Design review of the part built by this model. Coordinates are the model's own, in mm. Coordinates: 2 decimals unless noted, no trailing zeros. Loops run counter-clockwise (first coordinate to the right, second up) from the corner with the lowest first, then second, coordinate; pieces in that order, holes last. Notation, with made-up numbers: M 48,13.25 L 67,13.25 A29 ccw 67,40.25 Z; hole C 83,76 d4. An arc over 180 degrees is marked long. Write item = value, one per line. Start each with the question number.
```python
from build123d import *

# Parameters (mm, degrees)
SKETCH2_R           = 11.1125
BOSS_EXTRUDE1_DEPTH = 3.175
FILLET1_R           = 3
FILLET2_R           = 1


with BuildPart() as part:
    # Sketch2 → Boss-Extrude1 (new body)
    with BuildSketch(Plane.XY):
        with BuildLine():
            Line((-364.964629933, 19.05), (-397.035370067, 19.05))
            Line((-397.035370067, 19.05), (-397.035370067, -34.925))
            Line((-397.035370067, -34.925), (-520.207659615, -112.081032385))
            Line((-520.207659615, -112.081032385), (-530.464644327, -134.880029394))
            add(Edge.make_bspline(
                [(-457.420545856, -119.022880851), (-481.278146928, -107.716723517), (-513.288827873, -114.168548124), (-530.464644327, -134.880029394)],
                knots=[0.042886926, 0.042886926, 0.042886926, 0.042886926, 1, 1, 1, 1], degree=3))
            Line((-457.420545856, -119.022880851), (-364.964629933, -24.022670771))
            Line((-364.964629933, -24.022670771), (-364.964629933, 19.05))
        make_face()
        with Locations((-381, 0)):
            Circle(SKETCH2_R, mode=Mode.SUBTRACT)
    extrude(amount=BOSS_EXTRUDE1_DEPTH)

    # Fillet1
    fillet1_edges = [part.edges().sort_by_distance(p)[0] for p in [
        (-520.207659615, -112.081032385, 1.5875),
        (-397.035370067, -34.925, 1.5875),
        (-457.420545856, -119.022880851, 1.5875),
        (-364.964629933, -24.022670771, 1.5875),
        (-397.035370067, 19.05, 1.5875),
        (-364.964629933, 19.05, 1.5875),
    ]]
    fillet(fillet1_edges, radius=FILLET1_R)

    # Fillet2
    fillet2_edges = [part.edges().sort_by_distance(p)[0] for p in [
        (-530.464644327, -134.880029394, 1.5875),
    ]]
    fillet(fillet2_edges, radius=FILLET2_R)


solid = part.part
```
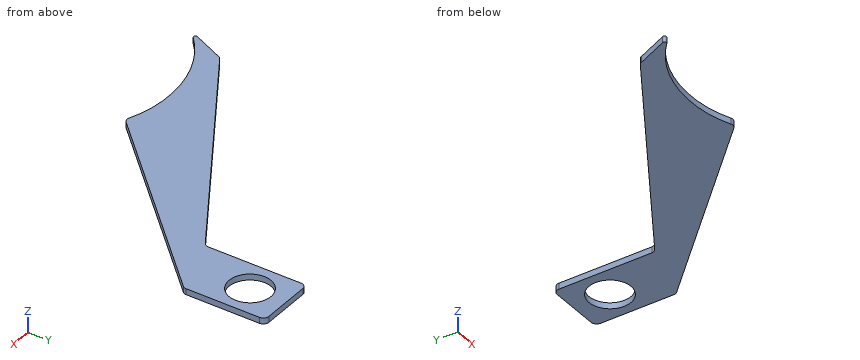
(1) To check wall thickness, follow L1, parallel to Y at x = -384, z = 2.5; L2, parallel to Y at x = -381, z = 2.2; L3, parallel to X at y = -18.5, z = 1.1. State the ranges of each line that lie inside material, in increasing order.
(2) Take a section at A-A (y = 0). State the section outline as (x, z) points (1 decimal).
(3) Take a section at C-C (y = -78.5). State the section outline as (x, z) points (3 decimals), plus the area to 3 significant figures.
(4) Insertion check: pin 1 (1 mm diameter, centred on x = -433.5, z = 2.5, fed in from +Y). The pin has a flat end and moves straight along its axis. Give the tip position at first contact, or say it passes through.
(5) Take a section at D-D (x = -427). State the section outline as (y, z) points (3 decimals), plus the area to 3 significant figures.
Results list:
q1.L1 = -43.58 to -10.7, 10.7 to 19.05
q1.L2 = -40.5 to -11.11, 11.11 to 19.05
q1.L3 = -397.04 to -364.96
q2.outline = M -397,0 L -392.1,0 L -392.1,3.2 L -397,3.2 Z; M -369.9,0 L -365,0 L -365,3.2 L -369.9,3.2 Z
q3.outline = M -466.599,0 L -417.983,0 L -417.983,3.175 L -466.599,3.175 Z
q3.area = 154 mm^2
q4.pin_1 = -57.45
q5.outline = M -87.765,0 L -53.695,0 L -53.695,3.175 L -87.765,3.175 Z
q5.area = 108 mm^2
